Source: CAD feature listing. Evaluate the final solid. Frame: model axes, mm. Give positions to 0.01 mm unless a question says otherwise; leave off trailing zeros. Order: outer loops, then holes, each group sorted by start corner. A loop starts at its lowest first (then second) coordinate and runs counter-clockwise, first axis right, second up. Notation, with made-up numbers: M 29,88.25 L 61,88.25 A24 ccw 61,124.25 Z; hole C 43,-31 d5. An arc over 180 degrees is marked long. Return JSON: item names as keys, results as strings.
from build123d import *

# Parameters (mm, degrees)
SKETCH1_W           = 1.5
SKETCH1_H           = 50
BOSS_EXTRUDE1_DEPTH = 93
SKETCH3_W           = 20
SKETCH3_H           = 11
SWITCH_DEPTH        = 2.5


with BuildPart() as part:
    # Sketch1 → Boss-Extrude1 (new body, symmetric)
    with BuildSketch(Plane(origin=(0, 0, 0), x_dir=(1, 0, 0), z_dir=(0, 1, 0))):
        Rectangle(SKETCH1_W, SKETCH1_H)
    extrude(amount=BOSS_EXTRUDE1_DEPTH, both=True)

    # Sketch3 → Switch (cut, through all)
    with BuildSketch(Plane.ZY.offset(0.75)):
        with Locations((0, 69.5)):
            Rectangle(SKETCH3_W, SKETCH3_H)
    extrude(amount=-SWITCH_DEPTH, mode=Mode.SUBTRACT)


solid = part.part
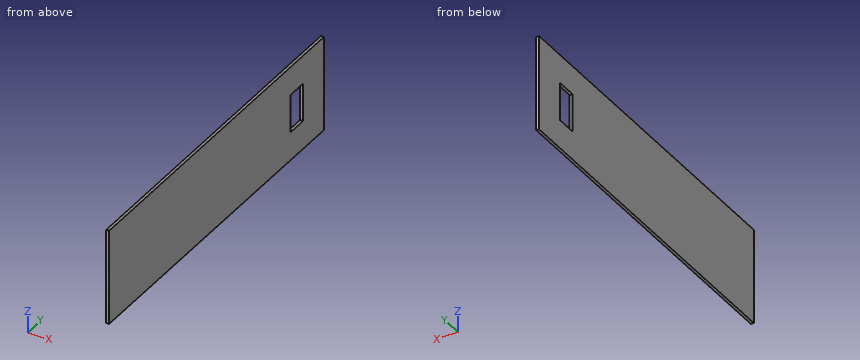
1. Section query A-A (y = 72.5). Return loops of the section in (x, z), then the cut area to 3 significant figures.
Evaluation:
{"outline": "M -0.75,-25 L 0.75,-25 L 0.75,-10 L -0.75,-10 Z; M -0.75,10 L 0.75,10 L 0.75,25 L -0.75,25 Z", "area": "45.0 mm^2"}
2. Section query B-B (x = -0.35). Return loops of the section in (y, z).
Evaluation:
{"outline": "M -93,-25 L 93,-25 L 93,25 L -93,25 Z; hole M 64,-10 L 75,-10 L 75,10 L 64,10 Z"}
3. Section query C-C (z = -2). Return loops of the section in (x, y).
Evaluation:
{"outline": "M -0.75,-93 L 0.75,-93 L 0.75,64 L -0.75,64 Z; M -0.75,75 L 0.75,75 L 0.75,93 L -0.75,93 Z"}
4. Ray query, probe 1 along Y at (x, z) = (-0.05, -4). Return the intervals inside material, ascending.
Evaluation:
{"probe 1": "y = -93 to 64, 75 to 93"}
